Job drawing, mm, ordinate dimensions from the low corner. One solid piece. Round coordinates to 2 decimals unless told otherwise and drop trailing zeros. Loops run counter-clockwise (first coordinate to the right, second up) from the corner with the lowest first, then second, coordinate; pieces in that order, holes last.
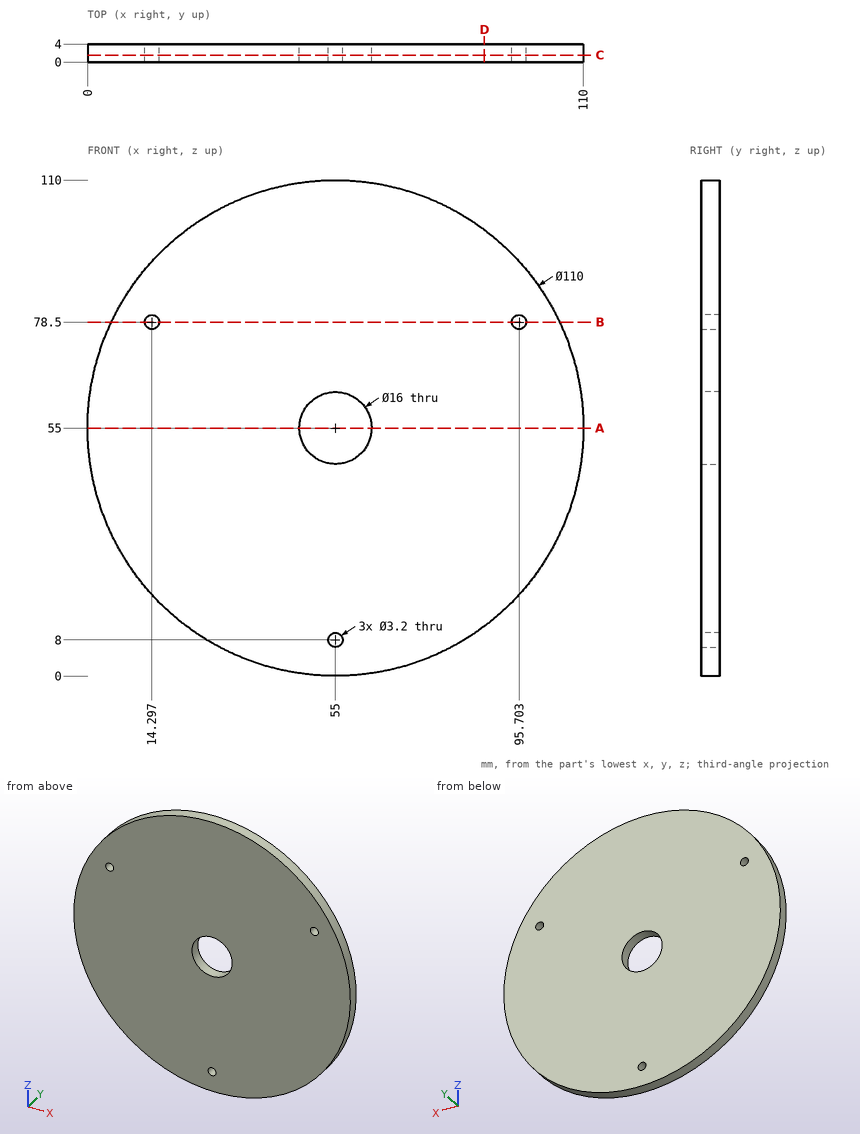
(1) Slice it at B-B on z = 78.5. List the corners of the cut face in (x, y).
Responses:
outline: (5.27, 0) - (12.7, 0) - (12.7, 4) - (5.27, 4) - close; (15.9, 0) - (94.1, 0) - (94.1, 4) - (15.9, 4) - close; (97.3, 0) - (104.73, 0) - (104.73, 4) - (97.3, 4) - close
(2) Probe line 1 (X direction, y = 3.05, z = 78.5); line 2 (Z direction, x = 50, y = 3.6) (1 decimal); line 3 (Z direction, x = 76, y = 1.4). List the from-to ranges inside material, lowest first.
Responses:
line 1: x = 5.27 to 12.7, 15.9 to 94.1, 97.3 to 104.73
line 2: z = 0.2 to 48.8, 61.2 to 109.8
line 3: z = 4.17 to 105.83
(3) Slice it at C-C on y = 1.55. List the corners of the cut face in (x, z).
Responses:
outline: circle Ø110 at (55, 55); hole circle Ø3.2 at (14.3, 78.5); hole circle Ø16 at (55, 55); hole circle Ø3.2 at (55, 8); hole circle Ø3.2 at (95.7, 78.5)
(4) Slice it at A-A on z = 55. List the corners of the cut face in (x, y), plus the area to 3 significant figures.
Responses:
outline: (0, 0) - (47, 0) - (47, 4) - (0, 4) - close; (63, 0) - (110, 0) - (110, 4) - (63, 4) - close
area: 376 mm2
(5) Pin check, flat tips, straight feed: P1, Ø5, axis at x = 40, z = 80.5, coming from the -Y side; P2, Ø2, axis at y = 3, z = 93.5, coming from the +X side. Stop position of each tip, or through.
Responses:
P1: stops at y = 0
P2: stops at x = 95.23
(6) Slice it at D-D on x = 88. List the corners of the cut face in (y, z).
Responses:
outline: (0, 11) - (4, 11) - (4, 99) - (0, 99) - close
